```python
from build123d import *

# Parameters (mm, degrees)
BASENUT_DEPTH = 16
DOMEFILLET_R  = 1


with BuildPart() as part:
    # BaseNutSke → BaseNut (new body)
    with BuildSketch(Plane(origin=(0, 0, 0), x_dir=(0, 0, -1), z_dir=(1, 0, 0))):
        Polygon((13.5, 7.794228634), (13.5, -7.794228634), (0, -15.588457268), (-13.5, -7.794228634), (-13.5, 7.794228634), (0, 15.588457268), align=None)
    extrude(amount=BASENUT_DEPTH)

    # DomeSke → Dome (revolve)
    with BuildSketch(Plane.XY, mode=Mode.PRIVATE) as dome_sk:
        with BuildLine():
            Line((26, 0), (24.4, 0))
            ThreePointArc((24.4, 0), (21.353910524, 7.353910524), (14, 10.4))
            Line((14, 10.4), (0, 10.4))
            Line((0, 10.4), (0, 12))
            Line((0, 12), (14, 12))
            ThreePointArc((14, 12), (22.485281374, 8.485281374), (26, 0))
        make_face()
    revolve(dome_sk.sketch.rotate(Axis((0, 0, 0), (1, 0, 0)), 180), axis=Axis((0, 0, 0), (1, 0, 0)))

    # Sketch4 → DoubleChamfer (revolve, cut)
    with BuildSketch(Plane.XY):
        Polygon((0, 13.5), (2.504809472, 17.838457268), (13.495190528, 17.838457268), (16, 13.5), (18, 13.5), (18, 28.5), (-2, 28.5), (-2, 13.5), align=None)
    revolve(axis=Axis((0, 0, 0), (1, 0, 0)), mode=Mode.SUBTRACT)

    # TapDriSke → TapDrill (revolve, cut)
    with BuildSketch(Plane.XY):
        Polygon((0, 8.75), (18.4, 8.75), (23.657530416, 0), (0, 0), align=None)
    revolve(axis=Axis((0, 0, 0), (1, 0, 0)), mode=Mode.SUBTRACT)

    # EndChamferSketch → EndChamfer (revolve, cut)
    with BuildSketch(Plane.XY, mode=Mode.PRIVATE) as endchamfer_sk:
        Polygon((-0.0746, 10), (0.0254, 10), (0.988185365, 8.625), (-0.0746, 8.625), align=None)
        Polygon((15.9746, 10), (16.1, 10), (16.1, 8.625), (15.011814635, 8.625), align=None)
    revolve(endchamfer_sk.sketch.rotate(Axis((0, 0, 0), (-1, 0, 0)), 90), axis=Axis((0, 0, 0), (-1, 0, 0)), mode=Mode.SUBTRACT)

    # DomeFillet
    domefillet_edges = [part.edges().sort_by_distance(p)[0] for p in [
        (16, 11.832159566, 0),
    ]]
    fillet(domefillet_edges, radius=DOMEFILLET_R)


solid = part.part
```
Here's how the part is built. I have some questions about the finished solid (model axes, mm). A direction names the side the tool comes from. Give positions to 0.01 mm unless a question says otherwise; leave off trailing zeros. Order: outer loops, then holes, each group sorted by start corner. A loop starts at its lowest first (then second) coordinate and runs counter-clockwise, first axis right, second up. Notation, with made-up numbers: (-21.5, 76.25) -> (27.5, 76.25) arc R7 cw to (27.5, 82.25) -> close; hole circle Ø1 at (-21.75, -7.75). An arc over 180 degrees is marked (long way). Use CSV: the item, a comma, the result in double quotes. Start each with the question number.
Item 1: I'm going to push flat-ended pins straight in: P1, Ø12, axis at x = 10.5, z = 5, coming from the -Y side; P2, Ø3, axis at y = -3, z = -9, coming from the +X side; P3, Ø1, axis at y = 2.5, z = 8.5, coming from the -X side. Where does each tip first touch, or does it pass through?
Item 2: On a 3-axis mill with a long thin cutter (end or side, diameter ignored), from which of +Z, -Z, +X, -X, +Y, -Y can I reach the whole of each face in a straight line? I mean faces 1 (the flat face through (16, -5, 12)), 2 (the conical face through (15.71, 7.03, 12.11)), 3 (the cylindrical face through (8.099, -6.944, -5.324)). Say none if no direction works.
Item 3: If I drill on probe 1 along Y at (x, z) = (0.05, 0); probe 2 along Z at (x, y) = (5.75, -1); probe 3 along Z at (x, y) = (12.25, 3), over which ranges is the centre line in solid material (lowest first)? Write a range as [from, to].
Item 4: Suppose I cut it at A-A (x = 9.5). List the corners of the cut face in (y, z) for me.
Item 5: Suppose I cut it at B-B (x = 22.5). List the corners of the cut face in (y, z) for me (1 decimal).
Answer block:
1,P1,"stops at y = -15.59"
1,P2,"stops at x = 22.96"
1,P3,"stops at x = 0.47"
2,face 1,"+X"
2,face 2,"+Z, +X, +Y"
2,face 3,"-X"
3,probe 1,"y = [-13.59, -9.96], [9.96, 13.59]"
3,probe 2,"z = [-13.5, -8.69], [8.69, 13.5]"
3,probe 3,"z = [-13.5, -8.22], [8.22, 13.5]"
4,outline,"(-15.59, 0) -> (-7.79, -13.5) -> (7.79, -13.5) -> (15.59, 0) -> (7.79, 13.5) -> (-7.79, 13.5) -> close; hole circle Ø17.5 at (0, 0)"
5,outline,"circle Ø16.9 at (0, 0); hole circle Ø12 at (0, 0)"
